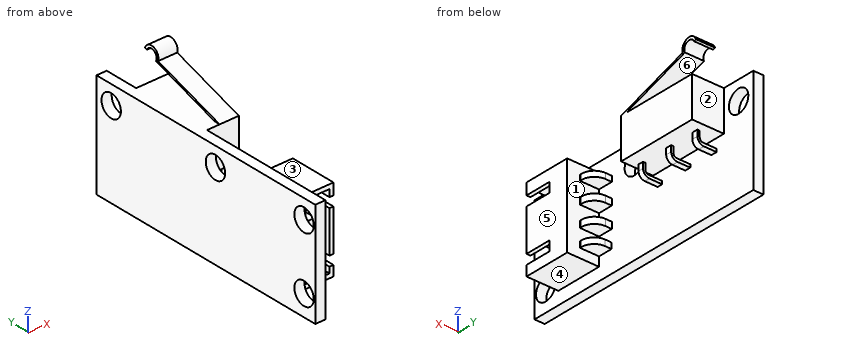
from build123d import *

# Parameters (mm, degrees)
SKETCH1_W           = 16.47
SKETCH1_H           = 39.44
BOSS_EXTRUDE1_DEPTH = 1.6
SKETCH2_W           = 6.3
SKETCH2_H           = 12.78
BOSS_EXTRUDE2_DEPTH = 5
SKETCH3_W           = 13
SKETCH3_H           = 7.33
BOSS_EXTRUDE3_DEPTH = 5
SKETCH4_W           = 0.849222168
SKETCH4_H           = 2.299281869
SKETCH4_W_2         = 0.996668432
SKETCH4_W_3         = 1.004572576
SKETCH4_W_4         = 0.915933819
SKETCH4_H_2         = 2.249002208
BOSS_EXTRUDE4_DEPTH = 3
SKETCH5_W           = 3.755878466
SKETCH5_H           = 11.665306642
CUT_EXTRUDE1_DEPTH  = 6
FILLET2_R           = 2
SKETCH6_W           = 1.024991321
SKETCH6_H           = 1.10945112
SKETCH6_H_2         = 1.02665626
SKETCH6_W_2         = 1.024991322
SKETCH6_H_3         = 1.059774204
SKETCH6_H_4         = 1.092892148
BOSS_EXTRUDE5_DEPTH = 5
SKETCH7_W           = 1.524548779
SKETCH7_H           = 4.1468753
CUT_EXTRUDE2_DEPTH  = 1
SKETCH8_W           = 1.935
SKETCH8_H           = 0.932620141
SKETCH8_H_2         = 0.892071439
SKETCH8_H_3         = 0.810974035
BOSS_EXTRUDE6_DEPTH = 3
FILLET3_R           = 1
CUT_EXTRUDE3_DEPTH  = 11
SKETCH10_R          = 1.75
CUT_EXTRUDE4_DEPTH  = 11
BOSS_EXTRUDE7_DEPTH = 3


with BuildPart() as part:
    # Sketch1 → Boss-Extrude1 (new body)
    with BuildSketch(Plane(origin=(0, 0, 0), x_dir=(0, 0, -1), z_dir=(1, 0, 0))):
        Rectangle(SKETCH1_W, SKETCH1_H)
    extrude(amount=BOSS_EXTRUDE1_DEPTH)

    # Sketch2 → Boss-Extrude2 (add)
    with BuildSketch(Plane(origin=(1.6, 0, 0), x_dir=(0, 0, -1), z_dir=(1, 0, 0))):
        with Locations((-5.085, 8.03)):
            Rectangle(SKETCH2_W, SKETCH2_H)
    extrude(amount=BOSS_EXTRUDE2_DEPTH)

    # Sketch3 → Boss-Extrude3 (add)
    with BuildSketch(Plane(origin=(1.6, 0, 0), x_dir=(0, 0, -1), z_dir=(1, 0, 0))):
        with Locations((-0.265, -11.755)):
            Rectangle(SKETCH3_W, SKETCH3_H)
    extrude(amount=BOSS_EXTRUDE3_DEPTH)

    # Sketch4 → Boss-Extrude4 (add)
    with BuildSketch(Plane(origin=(1.6, 0, 0), x_dir=(0, 0, -1), z_dir=(1, 0, 0))):
        with Locations((-4.874772316, -6.940359066)):
            Rectangle(SKETCH4_W, SKETCH4_H)
        with Locations((-1.665459639, -6.940359066)):
            Rectangle(SKETCH4_W_2, SKETCH4_H)
        with Locations((1.551129782, -6.940359066)):
            Rectangle(SKETCH4_W_3, SKETCH4_H)
        with Locations((4.343250619, -6.965498896)):
            Rectangle(SKETCH4_W_4, SKETCH4_H_2)
    extrude(amount=BOSS_EXTRUDE4_DEPTH)

    # Sketch5 → Cut-Extrude1 (cut)
    with BuildSketch(Plane(origin=(0, -15.42, 0), x_dir=(-1, 0, 0), z_dir=(0, -1, 0))):
        with Locations((-4.1, -0.265)):
            Rectangle(SKETCH5_W, SKETCH5_H)
    extrude(amount=-CUT_EXTRUDE1_DEPTH, mode=Mode.SUBTRACT)

    # Fillet2
    fillet2_edges = [part.edges().sort_by_distance(p)[0] for p in [
        (4.6, -5.790718131, 4.874772316),
        (4.6, -5.790718131, 1.665459639),
        (4.6, -5.790718131, -1.551129782),
        (4.6, -5.840997792, -4.343250618),
    ]]
    fillet(fillet2_edges, radius=FILLET2_R)

    # Sketch6 → Boss-Extrude5 (add)
    with BuildSketch(Plane(origin=(0, -9.42, 0), x_dir=(-1, 0, 0), z_dir=(0, -1, 0))):
        with Locations((-4.084273497, -4.083852883)):
            Rectangle(SKETCH6_W, SKETCH6_H)
        with Locations((-4.084273497, -1.715919896)):
            Rectangle(SKETCH6_W, SKETCH6_H_2)
        with Locations((-4.1, 1.14878225)):
            Rectangle(SKETCH6_W_2, SKETCH6_H_3)
        with Locations((-4.1, 3.467038322)):
            Rectangle(SKETCH6_W_2, SKETCH6_H_4)
    extrude(amount=BOSS_EXTRUDE5_DEPTH)

    # Sketch7 → Cut-Extrude2 (cut)
    with BuildSketch(Plane(origin=(6.6, 0, 0), x_dir=(0, 0, -1), z_dir=(1, 0, 0))):
        with Locations((-4.207178808, -13.34656235)):
            Rectangle(SKETCH7_W, SKETCH7_H)
        with Locations((3.868809321, -13.34656235)):
            Rectangle(SKETCH7_W, SKETCH7_H)
    extrude(amount=-CUT_EXTRUDE2_DEPTH, mode=Mode.SUBTRACT)

    # Sketch8 → Boss-Extrude6 (add)
    with BuildSketch(Plane(origin=(1.6, 0, 0), x_dir=(0, 0, -1), z_dir=(1, 0, 0))):
        with Locations((-0.9675, 12.634426175)):
            Rectangle(SKETCH8_W, SKETCH8_H)
        with Locations((-0.9675, 7.91050242)):
            Rectangle(SKETCH8_W, SKETCH8_H_2)
        with Locations((-0.9675, 2.8824634)):
            Rectangle(SKETCH8_W, SKETCH8_H_3)
    extrude(amount=BOSS_EXTRUDE6_DEPTH)

    # Fillet3
    fillet3_edges = [part.edges().sort_by_distance(p)[0] for p in [
        (4.6, 12.634426176, 0),
        (4.6, 7.910502419, 0),
        (4.6, 2.8824634, 0),
    ]]
    fillet(fillet3_edges, radius=FILLET3_R)

    # Sketch9 → Cut-Extrude3 (cut)
    with BuildSketch(Plane(origin=(0, 13.100736246, 0), x_dir=(1, 0, 0), z_dir=(0, 1, 0))):
        with BuildLine():
            Line((1.6, -0.469848577), (3.597144342, -0.469848577))
            add(Edge.make_bspline(
                [(3.597144342, -0.469848577), (4.148845696, -0.430996369), (4.233002481, -0.792491938), (4.243645389, -1.010671568)],
                knots=[0, 0, 0, 0, 1, 1, 1, 1], degree=3))
            Line((4.243645389, -1.010671568), (4.243645389, -1.935))
            Line((4.243645389, -1.935), (1.6, -1.935))
            Line((1.6, -1.935), (1.6, -0.469848577))
        make_face()
    extrude(amount=-CUT_EXTRUDE3_DEPTH, mode=Mode.SUBTRACT)

    # Sketch10 → Cut-Extrude4 (cut)
    with BuildSketch(Plane(origin=(1.6, 0, 0), x_dir=(0, 0, -1), z_dir=(1, 0, 0))):
        with Locations((-5.232585415, -1.723827663)):
            Circle(SKETCH10_R)
        with Locations((-5.232585415, 17.072870227)):
            Circle(SKETCH10_R)
        with Locations((-5.232585415, -17.69434278)):
            Circle(SKETCH10_R)
        with Locations((4.936201482, -17.69434278)):
            Circle(SKETCH10_R)
    extrude(amount=-CUT_EXTRUDE4_DEPTH, mode=Mode.SUBTRACT)

    # Sketch11 → Boss-Extrude7 (add)
    with BuildSketch(Plane(origin=(6.6, 0, 0), x_dir=(0, 0, -1), z_dir=(1, 0, 0))):
        with BuildLine():
            Line((-8.235, 1.64), (-11.930418499, 12.753922868))
            ThreePointArc((-11.930418499, 12.753922868), (-13.49815489, 13.539255516), (-12.712822243, 15.106991908))
            Line((-12.712822243, 15.106991908), (-12.58261695, 14.771125615))
            ThreePointArc((-12.58261695, 14.771125615), (-13.033453184, 13.523901114), (-11.761958985, 13.146906726))
            Line((-11.761958985, 13.146906726), (-8.235, 2.583341722))
            Line((-8.235, 2.583341722), (-8.235, 1.64))
        make_face()
    extrude(amount=-BOSS_EXTRUDE7_DEPTH)


solid = part.part
Could you check a few things on this model? Use its own coordinates, in mm. Face numbers are marked on the shaded views. A direction names the side the tool comes from. Coordinates: 2 decimals unless noted, no trailing zeros. Order: outer loops, then holes, each group sorted by start corner. A loop starts at its lowest first (then second) coordinate and runs counter-clockwise, first axis right, second up. Notation, with made-up numbers: (-36, 42) -> (-7, 42) arc R6 cw to (-7, 51) -> close; hole circle Ø7 at (66, 18.5). An arc over 180 degrees is marked (long way). One line per item, written item: value. Start each with the question number.
1) Imagine slicing it at A-A on x = 5.25. List the corners of the cut face in (y, z) for me (3 decimals).
2) I'm going to push flat-ended pins straight in: pin 1 (2 mm diameter, centred on x = 3.5, z = 1.5, fed in from -Y); pin 2 (1.1 mm diameter, centred on x = 4, y = -11, fed in from -Z) (3 decimals); pin 3 (1.1 mm diameter, centred on x = 3, y = -7, fed in from +Z). Where does each tip first touch, or does it pass through?
3) Imagine slicing it at D-D on y = 4.5. List the corners of the cut face in (x, z) for me (3 decimals).
4) We'd pull the mould along Z, two halves only. Please class the marked faces 4, 5 and 6: +Z half, -Z half, draft (parallel to the pull), parting line (faces both ways), or undercut.
5) Imagine slicing it at C-C on y = -16.5. List the corners of the cut face in (x, z) for me (1 decimal), plus the area to 3 significant figures.
6) Imagine slicing it at B-B on z = 7.5. List the corners of the cut face in (x, y) for me, plus the area to 3 significant figures.
7) If I drill on L1, parallel to Z at x = 2.25, y = -7.5; L2, parallel to Z at x = 5.25, y = -11.5 (3 decimals); L3, parallel to Y at x = 6, z = 6.25, over which ranges is the centre line in solid material (lowest first)? Write a range as [from, to].
8) Which directions (+Z, -Z, +X, -X, +Y, -Y) give clear straight access to the entire face, cutting with the end or side of a thin tool? Please do the marked faces 1, 2 and 3.
Answer list:
1. outline: (-15.42, -6.235) -> (-8.09, -6.235) -> (-8.09, 6.765) -> (-15.42, 6.765) -> (-15.42, 6.098) -> (-9.42, 6.098) -> (-9.42, -5.568) -> (-15.42, -5.568) -> close; (1.64, 1.935) -> (14.42, 1.935) -> (14.42, 8.235) -> (2.583, 8.235) -> (13.147, 11.762) arc R0.911 cw (long way) to (14.771, 12.583) -> (15.107, 12.713) arc R1.24 ccw to (12.754, 11.93) -> (1.64, 8.235) -> close
2. pin 1: stops at y = -14.42
2. pin 2: stops at z = -6.235
2. pin 3: stops at z = 5.3
3. outline: (0, -8.235) -> (1.6, -8.235) -> (1.6, 1.935) -> (6.6, 1.935) -> (6.6, 8.235) -> (0, 8.235) -> close; (3.6, 8.875) -> (6.6, 8.875) -> (6.6, 9.186) -> (3.6, 9.186) -> close
4. face 4: -Z half
4. face 5: draft
4. face 6: undercut
5. outline: (0, -8.2) -> (1.6, -8.2) -> (1.6, -6.2) -> (0, -6.2) -> close; (0, -3.7) -> (1.6, -3.7) -> (1.6, 4) -> (0, 4) -> close; (0, 6.5) -> (1.6, 6.5) -> (1.6, 8.2) -> (0, 8.2) -> close
5. area: 18.2 mm2
6. outline: (0, -19.72) -> (1.6, -19.72) -> (1.6, 1.64) -> (6.6, 1.64) -> (6.6, 14.42) -> (1.6, 14.42) -> (1.6, 19.72) -> (0, 19.72) -> close
6. area: 127 mm2
7. L1: z = [-4.8, -3.89], [-2.05, -1.05], [1.17, 2.16], [4.45, 5.3]
7. L2: z = [-6.235, -5.568], [6.098, 6.765]
7. L3: y = [-15.42, -8.09], [1.64, 14.42]
8. face 1: +X
8. face 2: -Z, +X, +Y
8. face 3: +Z, +X, -Y
